```python
from build123d import *

# Parameters (mm, degrees)
BOSS_EXTRUDE2_DEPTH = 14
SKETCH3_W           = 21
SKETCH3_H           = 54.5
SKETCH3_R           = 1.5
BOSS_EXTRUDE3_DEPTH = 2
SKETCH4_W           = 14
SKETCH4_H           = 54.5
CUT_EXTRUDE1_DEPTH  = 5
BOSS_EXTRUDE4_DEPTH = 5
BOSS_EXTRUDE6_DEPTH = 5
BOSS_EXTRUDE7_REACH = 10.7
SKETCH8_W           = 2
SKETCH8_H           = 4.5


with BuildPart() as part:
    # Sketch1 → Boss-Extrude2 (new body)
    with BuildSketch(Plane(origin=(0, 0, 0), x_dir=(1, 0, 0), z_dir=(0, 1, 0))):
        Polygon((0, 0), (-7, 0), (-21, 0), (-21, -54.5), (-13.577905098, -54.5), (0, -54.5), (0, -50.7), (-5.8, -50.7), (-19.8, -50.7), (-19.8, -41.9), (-5.8, -41.9), (0, -41.9), (0, -22.2), (-17, -22.2), (-17, -10), (-17, -3.5), (-10.5, -3.5), (-10.5, -10), (0, -10), align=None)
    extrude(amount=BOSS_EXTRUDE2_DEPTH)

    # Sketch3 → Boss-Extrude3 (add)
    with BuildSketch(Plane(origin=(0, 0, 0), x_dir=(1, 0, 0), z_dir=(0, 1, 0))):
        with Locations((-10.5, -27.25)):
            Rectangle(SKETCH3_W, SKETCH3_H)
        with Locations((-13.75, -6.75)):
            Circle(SKETCH3_R, mode=Mode.SUBTRACT)
    extrude(amount=-BOSS_EXTRUDE3_DEPTH)

    # Sketch4 → Cut-Extrude1 (cut)
    with BuildSketch(Plane(origin=(0, 14, 0), x_dir=(1, 0, 0), z_dir=(0, 1, 0))):
        with Locations((-14, -27.25)):
            Rectangle(SKETCH4_W, SKETCH4_H)
    extrude(amount=-CUT_EXTRUDE1_DEPTH, mode=Mode.SUBTRACT)

    # Sketch5 → Boss-Extrude4 (add)
    with BuildSketch(Plane.XY.offset(54.5)):
        Polygon((-12.3, -2), (0, -2), (0, 14), (-7, 14), (-7, 9), (-21, 9), (-21, -2), (-15.5, -2), align=None)
        Polygon((-7, 14), (0, 14), (0, 18.5), (-12.3, 18.5), (-12.3, 14), (-15.5, 14), (-15.5, 18.5), (-21, 18.5), (-21, 9), (-7, 9), align=None)
    extrude(amount=BOSS_EXTRUDE4_DEPTH)

    # Sketch7 → Boss-Extrude6 (add)
    with BuildSketch(Plane(origin=(0, 0, 0), x_dir=(-1, 0, 0), z_dir=(0, 0, -1))):
        Polygon((0, 18.5), (12.3, 18.5), (21, 18.5), (21, -2), (0, -2), align=None)
    extrude(amount=BOSS_EXTRUDE6_DEPTH)

    # Sketch8 → Boss-Extrude7 (add, up to next)
    with BuildSketch(Plane.ZY.offset(12.3), mode=Mode.PRIVATE) as boss_extrude7_sk1:
        with Locations((58.5, 16.25)):
            Rectangle(SKETCH8_W, SKETCH8_H)
    boss_extrude7_tool1 = extrude(boss_extrude7_sk1.sketch, amount=BOSS_EXTRUDE7_REACH, mode=Mode.PRIVATE) - part.part
    add(boss_extrude7_tool1.solids().sort_by_distance((-12.3, 16.25, 58.5))[0])


solid = part.part
```
Geometry: final body of the model. Coordinates: model frame, mm. A direction names the side the tool comes from. Round coordinates to 2 decimals unless told otherwise and drop trailing zeros. Write each loop counter-clockwise with the first axis right and the second up, starting at its lowest first coordinate (ties: lowest second). Pieces come first, ordered by that corner, then holes. Notation, with made-up numbers: (7, -28) -> (25, -28) arc R24 ccw to (25, 1) -> close; hole circle Ø9 at (-5, -12.75). An arc over 180 degrees is marked (long way). Return JSON: item names as keys, results as strings.
Q1. Section A-A on x = -13.75. Return the cut outline in (y, z).
From the geometry:
{"outline": "(-2, -5) -> (18.5, -5) -> (18.5, 0) -> (9, 0) -> (9, 3.5) -> (0, 3.5) -> (0, 5.25) -> (-2, 5.25) -> close; (-2, 8.25) -> (0, 8.25) -> (0, 22.2) -> (9, 22.2) -> (9, 41.9) -> (0, 41.9) -> (0, 50.7) -> (9, 50.7) -> (9, 54.5) -> (14, 54.5) -> (14, 57.5) -> (18.5, 57.5) -> (18.5, 59.5) -> (-2, 59.5) -> close"}
Q2. First-contact query: pin 1 Ø2.5 at (y, z) = (3, 13.5) entering from +X; pin 2 Ø5.5 at (y, z) = (12, 5.5) entering from -X. Flat tips, straight axial feed; report the tip coordinate or a pass-through.
From the geometry:
{"pin 1": "x = -17", "pin 2": "x = -7"}
Q3. Section D-D on y = 6.5. Return the cut outline in (x, z).
From the geometry:
{"outline": "(-21, -5) -> (0, -5) -> (0, 10) -> (-10.5, 10) -> (-10.5, 3.5) -> (-17, 3.5) -> (-17, 22.2) -> (0, 22.2) -> (0, 41.9) -> (-19.8, 41.9) -> (-19.8, 50.7) -> (0, 50.7) -> (0, 59.5) -> (-21, 59.5) -> close"}
Q4. Ray query, line 1 (Z direction, x = -4.5, y = 5.25); line 2 (Z direction, x = -14.25, y = 4.5); line 3 (Z direction, x = -13.75, y = -0.4). Return the intervals inside material, ascending.
From the geometry:
{"line 1": "-5 to 10, 22.2 to 41.9, 50.7 to 59.5", "line 2": "-5 to 3.5, 22.2 to 41.9, 50.7 to 59.5", "line 3": "-5 to 5.25, 8.25 to 59.5"}
Q5. Section C-C on x = -9.5. Return the cut outline in (y, z).
From the geometry:
{"outline": "(-2, -5) -> (18.5, -5) -> (18.5, 0) -> (9, 0) -> (9, 10) -> (0, 10) -> (0, 22.2) -> (9, 22.2) -> (9, 41.9) -> (0, 41.9) -> (0, 50.7) -> (9, 50.7) -> (9, 54.5) -> (18.5, 54.5) -> (18.5, 59.5) -> (-2, 59.5) -> close"}
Q6. Set-up query: faces 1 (the flat face through (-4, 14, 32)), 2 (the flat face through (-7, 12, 53)), 3 (the flat face through (-8, 5, 22.2)), 4 (the flat face through (-17, 4, 13)). Return all of +Z, -Z, +X, -X, +Y, -Y with unobstructed straight access to the full face (end or side cutting, diameter ignored); none if empty.
From the geometry:
{"face 1": "+X, -X, +Y", "face 2": "-X, +Y", "face 3": "+X, +Y", "face 4": "+Y"}
Q7. Mould query, pull axis X, two halves, no side actions, for faces 5 (the flat face through (-7, 12, 5)), 6 (the flat face through (-4, 14, 5)), 7 (the cylindrical face through (-15.25, -0.99, 6.68)), 8 (the flat face through (-15.5, 16, 56)). Classes: +X half, -X half, draft (parallel to the pull), parting line (faces both ways), or undercut.
From the geometry:
{"face 5": "-X half", "face 6": "draft", "face 7": "undercut", "face 8": "undercut"}
Q8. Section B-B on z = 6.75. Return the cut outline in (x, y), and give its area (4 significant figures).
From the geometry:
{"outline": "(-21, -2) -> (-15.25, -2) -> (-15.25, 0) -> (-17, 0) -> (-17, 9) -> (-21, 9) -> close; (-12.25, -2) -> (0, -2) -> (0, 14) -> (-7, 14) -> (-7, 9) -> (-10.5, 9) -> (-10.5, 0) -> (-12.25, 0) -> close", "area": "201.5 mm2"}
